Job drawing, mm, ordinate dimensions from the low corner. One solid piece. Round coordinates to 2 decimals unless told otherwise and drop trailing zeros. Write each loop counter-clockwise with the first axis right and the second up, starting at its lowest first coordinate (ties: lowest second). Pieces come first, ordered by that corner, then holes.
1) Saw through at D-D on y = 5.5. Write the cut outline in (x, z).
2) Drill centre lines: L1, parallel to Y at x = 5.25, z = 7.25; L2, parallel to X at y = 1.75, z = 6.5 (1 decimal); L3, parallel to X at y = 3, z = 10. Where is each one in solid material? Low to high.
3) Saw through at A-A on x = 5.25. Write the cut outline in (y, z).
4) Flat gauge pins, fed straight in: pin 1 (1.5 mm diameter, centred on x = 1, z = 3.5, fed in from +Y); pin 2 (3 mm diameter, centred on x = 5.25, y = 3.14, fed in from +Z). Where does each tip first touch, or does it go through?
5) Pull direction Y, two halves, no side cores. Call the marked faces 1, 2 and 3: +Y half, -Y half, draft (parallel to the pull), parting line (faces both ways), or undercut.
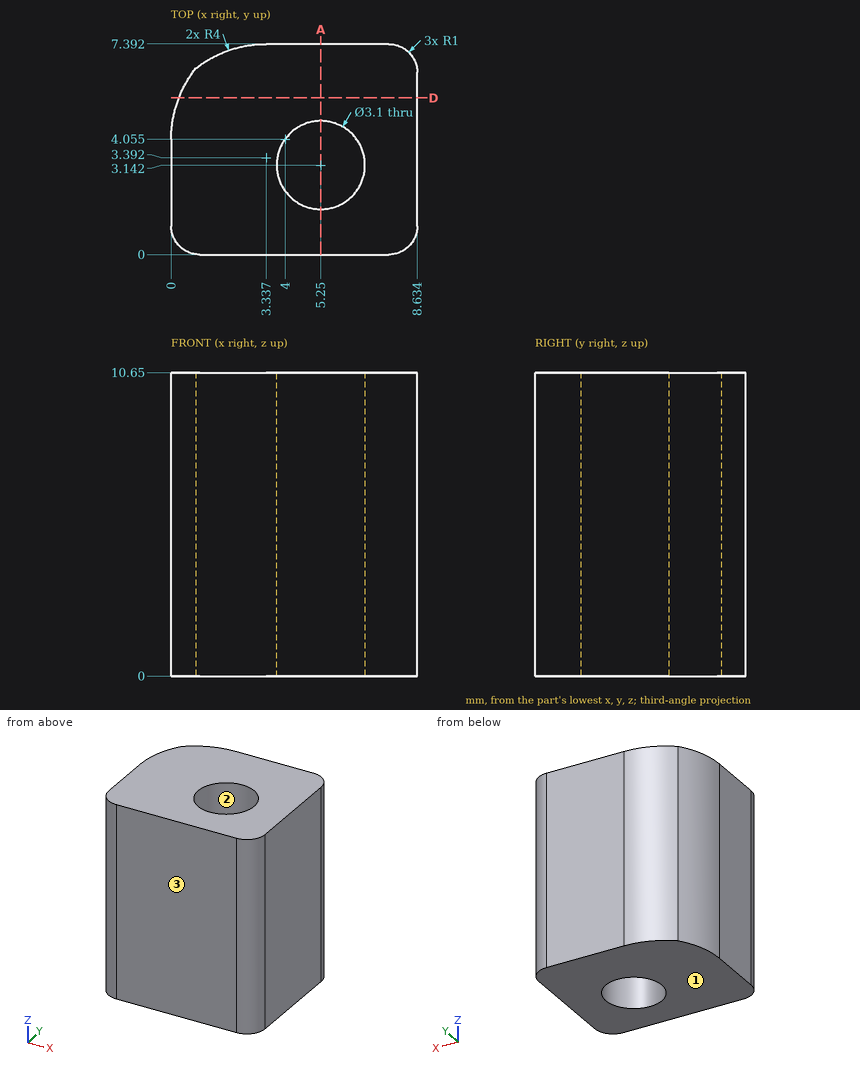
Completed:
1. outline: (0.27, 0) - (8.63, 0) - (8.63, 10.65) - (0.27, 10.65) - close
2. L1: y = 0 to 1.59, 4.69 to 7.39
2. L2: x = 0 to 4.6, 5.9 to 8.6
2. L3: x = 0 to 3.71, 6.79 to 8.63
3. outline: (0, 0) - (1.59, 0) - (1.59, 10.65) - (0, 10.65) - close; (4.69, 0) - (7.39, 0) - (7.39, 10.65) - (4.69, 10.65) - close
4. pin 1: stops at y = 7.06
4. pin 2: passes through
5. face 1: draft
5. face 2: undercut
5. face 3: -Y half
